The model under review builds one solid part; all positions refer to its coordinate system, in mm. Coordinates: 2 decimals unless noted, no trailing zeros. Order: outer loops, then holes, each group sorted by start corner. A loop starts at its lowest first (then second) coordinate and runs counter-clockwise, first axis right, second up.
```python
from build123d import *

# Parameters (mm, degrees)
SKETCH1_R           = 90
BOSS_EXTRUDE1_DEPTH = 0.5
SKETCH3_W           = 31.4086089
SKETCH3_H           = 76.2
CUT_EXTRUDE2_DEPTH  = 1


with BuildPart() as part:
    # Sketch1 → Boss-Extrude1 (new body)
    with BuildSketch(Plane(origin=(0, 0, 0), x_dir=(1, 0, 0), z_dir=(0, 1, 0))):
        Circle(SKETCH1_R)
    extrude(amount=BOSS_EXTRUDE1_DEPTH)

    # Sketch3 → Cut-Extrude2 (cut)
    with BuildSketch(Plane(origin=(0, 0.5, 0), x_dir=(1, 0, 0), z_dir=(0, 1, 0))):
        with Locations((64.29569555, 0)):
            Rectangle(SKETCH3_W, SKETCH3_H)
        with Locations((-63.00534762, 0)):
            Rectangle(SKETCH3_W, SKETCH3_H)
    extrude(amount=-CUT_EXTRUDE2_DEPTH, mode=Mode.SUBTRACT)


solid = part.part
```
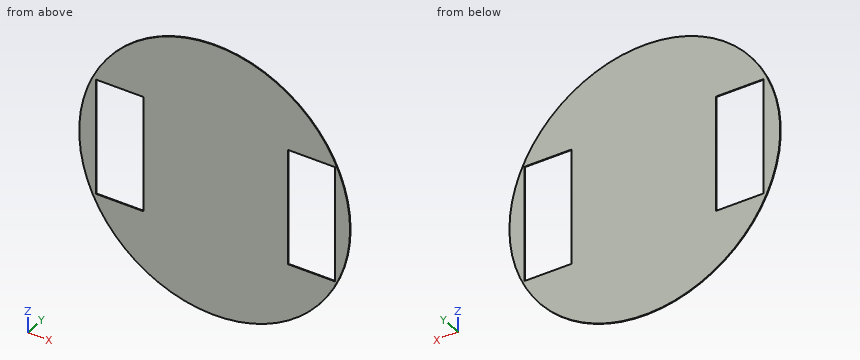
(1) Wall thickness on probe 1 along X at (y, z) = (0.3, -10); probe 2 along X at (y, z) = (0.3, -24.5); probe 3 along Z at (x, y) = (27.5, 0.3): over which ranges is each line inside the solid? List them lowest first.
A:
probe 1: x = -89.44 to -78.71, -47.3 to 48.59, 80 to 89.44
probe 2: x = -86.6 to -78.71, -47.3 to 48.59, 80 to 86.6
probe 3: z = -85.7 to 85.7
(2) We need section B-B, the plane y = 0.25. Write out the cut boundary in (x, z).
A:
outline: circle Ø180 at (0, 0); hole (-78.71, -38.1) - (-47.3, -38.1) - (-47.3, 38.1) - (-78.71, 38.1) - close; hole (48.59, -38.1) - (80, -38.1) - (80, 38.1) - (48.59, 38.1) - close
(3) We need section A-A, the plane z = 0. Write out the cut boundary in (x, y).
A:
outline: (-90, 0) - (-78.71, 0) - (-78.71, 0.5) - (-90, 0.5) - close; (-47.3, 0) - (48.59, 0) - (48.59, 0.5) - (-47.3, 0.5) - close; (80, 0) - (90, 0) - (90, 0.5) - (80, 0.5) - close
(4) We need section D-D, the plane z = -54. Write out the cut boundary in (x, y), and give its area (3 significant figures).
A:
outline: (-72, 0) - (72, 0) - (72, 0.5) - (-72, 0.5) - close
area: 72.0 mm2
(5) We need section C-C, the plane x = 28.5. Write out the cut boundary in (y, z).
A:
outline: (0, -85.37) - (0.5, -85.37) - (0.5, 85.37) - (0, 85.37) - close
